Design review of the part built by this model. Coordinates are the model's own, in mm. A direction names the side the tool comes from. Round coordinates to 2 decimals unless told otherwise and drop trailing zeros. Write each loop counter-clockwise with the first axis right and the second up, starting at its lowest first coordinate (ties: lowest second). Pieces come first, ordered by that corner, then holes. Notation, with made-up numbers: (17.25, 65.5) -> (23.25, 65.5) arc R22 cw to (23.25, 91.5) -> close; hole circle Ø3 at (-9.75, 4.5). An arc over 180 degrees is marked (long way). One line per question, with ' | ' between items. Start each with the question number.
1) Consider section B-B (z = -54). Give the boundary of the cut face in (x, y), then the cut area to 3 significant figures.
2) Consider section C-C (x = -27). Give the boundary of the cut face in (y, z).
3) Mouldability with a two-part tool opening along X and no side actions: class faces 3 (the cylindrical face through (-3.917, -0.917, -50.089)), 4 (the cylindrical face through (-1.738, 1.215, -50.089)), 5 (the flat face through (-2.87, -16.83, 0)) as +X half, -X half, draft (parallel to the pull), parting line (faces both ways), or undercut.
4) Consider section D-D (x = -10.5). Give the boundary of the cut face in (y, z), then the cut area to 3 significant figures.
5) For faces 1 (the flat face through (-31.75, -26, -52)), 2 (the flat face through (-28.702, -25, -52)), list the 3-axis set-ups (+Z, -Z, +X, -X, +Y, -Y) from which the entire face can be reached by the end or side of a thin tool; tool diameter is ignored.
6) Consider section A-A (y = -4.5). Give the boundary of the cut face in (x, z), then the cut area to 3 significant figures.
7) For probe 1 along X at (y, z) = (-16, -35.5); probe 2 along Y at (x, z) = (-18, -47.5); probe 3 along X at (y, z) = (-1, -72), list the stretches that pass through material, from the lowest coordinate up.
Autodesk Inventor part; units mm, degrees
ref_plane "YZ Plane" through (0, 0, 0) normal (1, 0, 0) x (0, 1, 0)
ref_plane "XZ Plane" through (0, 0, 0) normal (0, 1, 0) x (-1, 0, 0)
ref_plane "XY Plane" through (0, 0, 0) normal (0, 0, 1) x (1, 0, 0)
sketch "Sketch1" plane through (0, 0, 0) normal (0, 1, 0) x (-1, 0, 0)
  line L0 (0, 0) -> (31.75, 0)
  line L1 (31.75, 0) -> (31.75, -101.6)
  line L2 (31.75, -101.6) -> (0, -101.6)
  line L3 (0, -101.6) -> (0, 0)
  dimension "d0" = 31.75
  dimension "d1" = 101.6
extrude "Plate1" add sketch "Sketch1" along normal blind 3.048
sketch "Sketch2" plane through (-3.048, 3.048, 0) normal (1, 0, 0) x (0, 1, 0)
  line L0 (0, -101.6) -> (0, 0)
  line L1 (0, 0) -> (-50.8, 0)
  line L2 (-50.8, 0) -> (-50.8, -101.6)
  line L3 (-50.8, -101.6) -> (0, -101.6)
edge flange "Flange1" height 50.8 angle 90 thickness 3.048 bend radius 3.048 thickness toward (1, 0, 0) relief tear relief width 3.048 relief depth 1.524 corner gap 3.048 corner form 0 edges at (0, 0, -50.8) (-31.75, 0, -50.8) wall of the first edge with corners at (-3.048, 3.048, -101.6) (-3.048, 3.048, 0) (-3.048, -47.752, 0) (-3.048, -47.752, -101.6)
bend "Bend1"
corner "Corner1"
equation "\"d3\" = BendReliefWidth"
equation "\"d4\" = BendReliefDepth"
equation "\"d5\" = MinimumRemnant"
equation "\"d6\" = BendRadius"
equation "\"d9\" = BendRadius"
equation "\"d10\" = CornerReliefSize"
equation "\"d11\" = GapSize"
equation "\"d12\" = JacobiRadiusSize"
equation "\"BendRadius\" = Thickness"
equation "\"BendReliefWidth\" = Thickness"
equation "\"BendReliefDepth\" = 0.5 * Thickness"
equation "\"CornerReliefSize\" = 4 * Thickness"
equation "\"MinimumRemnant\" = 2 * Thickness"
equation "\"TransitionRadius\" = BendRadius"
equation "\"JacobiRadiusSize\" = BendRadius"
equation "\"GapSize\" = Thickness"
equation "\"d2\" = BendRadius"
properties part number "aFrameBrace1"
From the geometry:
1) outline: (-31.75, -47.75) -> (-28.7, -47.75) -> (-28.7, -3.05) arc R3.05 cw to (-25.65, 0) -> (-6.1, 0) arc R3.05 cw to (-3.05, -3.05) -> (-3.05, -47.75) -> (0, -47.75) -> (0, -3.05) arc R6.1 ccw to (-6.1, 3.05) -> (-25.65, 3.05) arc R6.1 ccw to (-31.75, -3.05) -> close | area: 376 mm2
2) outline: (-0.31, -101.6) -> (2.9, -101.6) -> (2.9, 0) -> (-0.31, 0) -> close
3) face 3: undercut | face 4: +X half | face 5: draft
4) outline: (0, -101.6) -> (3.05, -101.6) -> (3.05, 0) -> (0, 0) -> close | area: 310 mm2
5) face 1: +Z, -Z, -X, +Y, -Y | face 2: +Z, -Z, -Y
6) outline: (-31.75, -101.6) -> (-28.7, -101.6) -> (-28.7, 0) -> (-31.75, 0) -> close; (-3.05, -101.6) -> (0, -101.6) -> (0, 0) -> (-3.05, 0) -> close | area: 619 mm2
7) probe 1: x = -31.75 to -28.7, -3.05 to 0 | probe 2: y = 0 to 3.05 | probe 3: x = -31.4 to -27.91, -3.84 to -0.35
